The listing builds one solid part. Answer for the finished solid, in the listing's coordinates (mm). A direction names the side the tool comes from. Round coordinates to 2 decimals unless told otherwise and drop trailing zeros. Order: outer loops, then holes, each group sorted by start corner. A loop starts at its lowest first (then second) coordinate and runs counter-clockwise, first axis right, second up. Notation, with made-up numbers: (28, 68) - (86, 68) arc R18 ccw to (86, 93) - close; hole circle Ø5 at (-8, 68.5). An arc over 180 degrees is marked (long way). One line per item, written item: value. Start each with the question number.
1. A tool of negligible diameter and unlimited length cuts with its end or side. For faces 1 (the flat face through (32, 16, -7)), 2 (the flat face through (-1, 76, 5)), 3 (the flat face through (32, 96, 0)), from which of +Z, -Z, +X, -X, +Y, -Y can it reach the whole face along a straight path? Write none if from no direction.
2. Section B-B, the plane x = -10 is taken. Give the vertices of the cut face in (y, z), then the cut area to 3 significant figures.
3. Straight lines are drawn through the part: line 1 (Y direction, x = -40.5, z = 1.75); line 2 (X direction, y = -16, z = 3.75); line 3 (X direction, y = -56, z = -1.25). For each, find the intervals that lie inside material, in ascending order.
4. Flat-ended cylindrical pins translate along their axes: P1, Ø7.5, axis at y = 40.5, z = -4, coming from the +X side; P2, Ø1.5, axis at x = -31.5, y = -78.5, coming from the +Z side; P3, Ø2.5, axis at x = -32.5, z = 1.5, coming from the +Y side. Find the tip coordinate at first contact, or state that the pin passes through.
5. Section C-C, the plane y = 28 is taken. Give the vertices of the cut face in (x, z), then the cut area to 3 significant figures.
6. For a pull along Y with two mould halves and no side action, classify faces 4 (the flat face through (30, 14, -3)), 5 (the flat face through (-1, 9, 2)), 6 (the flat face through (-33, 120, -3)) as released by +Y, released by -Y, zero draft, split by the parting line, or undercut.
7. Section A-A, the plane z = -3.25 is taken. Give the vertices of the cut face in (x, y).
from build123d import *

# Parameters (mm, degrees)
F1_DEPTH = 7
F2_W     = 180
F2_H     = 5
F3_DEPTH = 5
F4_W     = 5.000001
F4_H     = 210
F4_W_2   = 5
F5_DEPTH = 7


with BuildPart() as f1:
    # F0 (on Top) → F1 (new body)
    with BuildSketch(Plane.XY):
        Polygon((94.104588, 118.803262), (-93.895412, 118.803262), (-93.895412, -91.196738), (-88.895412, -91.196738), (-88.895412, 113.803262), (89.104588, 113.803262), (89.104588, -91.196738), (94.104588, -91.196738), align=None)
    extrude(amount=F1_DEPTH)

    # F2 (on Top) → F3 (join)
    with BuildSketch(Plane.XY):
        with Locations((0.104588, 75.474764)):
            Rectangle(F2_W, F2_H)
        with Locations((0.104588, 11.5)):
            Rectangle(F2_W, F2_H)
        with Locations((0.104588, -59.49998)):
            Rectangle(F2_W, F2_H)
    extrude(amount=F3_DEPTH)

    # F4 (on Top) → F5 (join)
    with BuildSketch(Plane.XY):
        with Locations((-32.5, 15)):
            Rectangle(F4_W, F4_H)
        with Locations((32.5, 15)):
            Rectangle(F4_W_2, F4_H)
    extrude(amount=-F5_DEPTH)


solid = f1.part
Answer list:
1. face 1: -Z, +X, -X, +Y, -Y
1. face 2: +Z, -Y
1. face 3: +Z
2. outline: (-62, 0) - (-57, 0) - (-57, 5) - (-62, 5) - close; (9, 0) - (14, 0) - (14, 5) - (9, 5) - close; (72.97, 0) - (77.97, 0) - (77.97, 5) - (72.97, 5) - close; (113.8, 0) - (118.8, 0) - (118.8, 7) - (113.8, 7) - close
2. area: 110 mm²
3. line 1: y = -62 to -57, 9 to 14, 72.97 to 77.97, 113.8 to 118.8
3. line 2: x = -93.9 to -88.9, 89.1 to 94.1
3. line 3: x = -35 to -30, 30 to 35
4. P1: stops at x = 35
4. P2: stops at z = 0
4. P3: stops at y = 118.8
5. outline: (-93.9, 0) - (-88.9, 0) - (-88.9, 7) - (-93.9, 7) - close; (-35, -7) - (-30, -7) - (-30, 0) - (-35, 0) - close; (30, -7) - (35, -7) - (35, 0) - (30, 0) - close; (89.1, 0) - (94.1, 0) - (94.1, 7) - (89.1, 7) - close
5. area: 140 mm²
6. face 4: zero draft
6. face 5: undercut
6. face 6: released by +Y
7. outline: (-35, -90) - (-30, -90) - (-30, 120) - (-35, 120) - close; (30, -90) - (35, -90) - (35, 120) - (30, 120) - close
